Autodesk Inventor part; units mm, degrees
ref_plane "YZ Plane" through (0, 0, 0) normal (1, 0, 0) x (0, 1, 0)
ref_plane "XZ Plane" through (0, 0, 0) normal (0, 1, 0) x (-1, 0, 0)
ref_plane "XY Plane" through (0, 0, 0) normal (0, 0, 1) x (1, 0, 0)
sketch "Sketch1" plane through (0, 0, 0) normal (0, 1, 0) x (-1, 0, 0)
  line L0 (0, 0) -> (0, -8)
  circle A0 centre (0, -8) radius 3
  line L1 (0, 0) -> (0, 8)
  circle A1 centre (0, 8) radius 2.5
  circle A2 centre (0, 8) radius 3.75
  circle A3 centre (0, -8) radius 3.75
  line L2 (3.75, 8) -> (3.75, -8)
  line L3 (-3.75, 8) -> (-3.75, -8)
  line L4 (3.75, 4.25) -> (-3.75, 4.25)
  line L5 (3.75, -4.25) -> (-3.75, -4.25)
  point P0 (-2.6582, -4.25)
  dimension "d0" = 8
  dimension "d1" = 6
  dimension "d2" = 8
  dimension "d3" = 5
  dimension "d4" = 7.5
  dimension "d5" = 7.5
  dimension "d6" = 8.5
extrude "Extrusion1" add sketch "Sketch1" along normal blind 5 contours L1 L4 L2 L5 L0 | L0 L5 L3 L4 L1 | L4 L3 A2 | A2 | A2 L2 L4
sketch "Sketch2" plane through (3.75, 0, -4.25) normal (0, 0, -1) x (-1, 0, 0)
  line L0 (0, 5) -> (7.5, 5)
  line L1 (0, 0) -> (7.5, 0)
  line L2 (7.5, 0) -> (7.5, 5)
  line L3 (7.5, 5) -> (0, 5)
  line L4 (0, 5) -> (0, 0)
  line L5 (0, 0) -> (7.5, 5) construction
  line L6 (7.5, 0) -> (0, 5) construction
  circle A0 centre (3.75, 2.5) radius 1.5
  line L7 (1.25, 1.5) -> (6.25, 1.5)
  line L8 (6.25, 1.5) -> (6.25, 3.5)
  line L9 (6.25, 3.5) -> (1.25, 3.5)
  line L10 (1.25, 3.5) -> (1.25, 1.5)
  line L11 (1.25, 1.5) -> (6.25, 3.5) construction
  line L12 (6.25, 1.5) -> (1.25, 3.5) construction
  point P0 (3.75, 0)
  point P1 (4.868, 1.5)
  point P2 (2.632, 1.5)
  point P3 (2.632, 3.5)
  point P4 (4.868, 3.5)
  dimension "d9" = 3
  dimension "d10" = 5
  dimension "d11" = 2
extrude "Extrusion2" cut sketch "Sketch2" against normal blind 8.5
sketch "Sketch3" plane through (3.75, 0, 8) normal (1, 0, 0) x (0, 0, -1)
  line L0 (0, 0) -> (0, 5)
  circle A0 centre (0, 2.5) radius 1.5
  point P0 (8, 0)
  dimension "d14" = 3
extrude "Extrusion3" add sketch "Sketch3" along normal mid plane 1.5
sketch "Sketch4" plane through (4.5, 2.5, 8) normal (1, 0, 0) x (0, 0, -1)
  line L0 (0, -2.5) -> (0, 2.5)
  circle A0 centre (0, 0) radius 1
  point P0 (8, -2.5)
  dimension "d17" = 2
extrude "Extrusion4" cut sketch "Sketch4" against normal blind 3.2625
properties part number "Link_InsideV3"
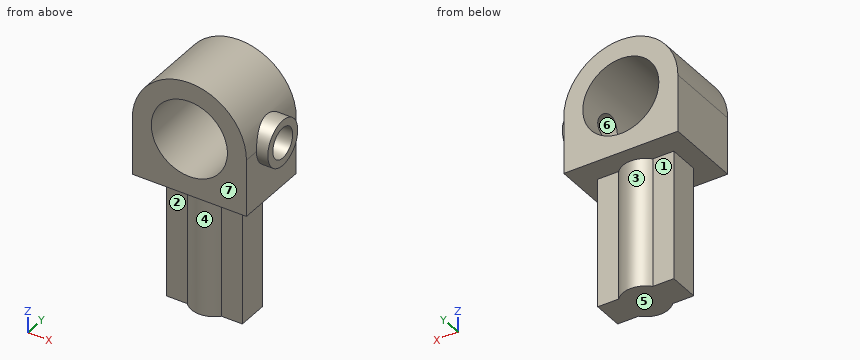
Input: part model. Units: mm. Frame: model coordinates. Face numbers are marked on the shaded views. A direction names the side the tool comes from. Give positions to 0.01 mm unless a question says otherwise; leave off trailing zeros. Order: outer loops, then holes, each group sorted by start corner. A loop starts at its lowest first (then second) coordinate and runs counter-clockwise, first axis right, second up.
1. Draft query along Z for the marked faces 5, 6 and 7. Return one class per face: released by +Z, released by -Z, zero draft, split by the parting line, or undercut.
Computed:
face 5: released by -Z
face 6: undercut
face 7: zero draft
2. Pin query (flat end, axial travel): pin 1 Ø1.1 at (x, z) = (-2, -2) entering from +Y; pin 2 Ø1 at (y, z) = (2, 0.5) entering from -X; pin 3 Ø0.6 at (y, z) = (3, 2) entering from +X. Return the tip coordinate at first contact, or that it passes through.
Computed:
pin 1: stops at y = 3.5
pin 2: stops at x = -2.5
pin 3: stops at x = 2.5
3. Cut plane A-A (x = 0). Return loops of the section in (y, z), and give its area (3 significant figures).
Computed:
outline: (0, 4.25) - (1, 4.25) - (1, -4.25) - (4, -4.25) - (4, 4.25) - (5, 4.25) - (5, 5.5) - (0, 5.5) - close; (0, 10.5) - (5, 10.5) - (5, 11.75) - (0, 11.75) - close
area: 38.0 mm2
4. Cut plane D-D (y = 2.5). Return loops of the section in (x, z), and give its area (3 significant figures).
Computed:
outline: (-3.75, 4.25) - (-2.5, 4.25) - (-2.5, -4.25) - (2.5, -4.25) - (2.5, 4.25) - (3.75, 4.25) - (3.75, 6.5) - (4.5, 6.5) - (4.5, 7) - (2.29, 7) arc R2.5 cw (long way) to (2.29, 9) - (4.5, 9) - (4.5, 9.5) - (3.44, 9.5) arc R3.75 ccw to (-3.75, 8) - close
area: 71.3 mm2
5. Cut plane B-B (z = 2.5). Return loops of the section in (x, y), and give its area (3 significant figures).
Computed:
outline: (-2.5, 1.5) - (-1.12, 1.5) arc R1.5 ccw to (1.12, 1.5) - (2.5, 1.5) - (2.5, 3.5) - (1.12, 3.5) arc R1.5 ccw to (-1.12, 3.5) - (-2.5, 3.5) - close
area: 11.5 mm2
6. Cut plane C-C (x = 3). Return loops of the section in (y, z), and give its area (3 significant figures).
Computed:
outline: (0, 4.25) - (5, 4.25) - (5, 10.25) - (0, 10.25) - close; hole circle Ø2 at (2.5, 8)
area: 26.9 mm2
7. Line query: probe 1 along Z at (x, y) = (0, 2.55); probe 2 along Y at (x, z) = (3.1, 8); probe 3 along Z at (x, y) = (4.05, 2.5). Output: solid intervals per line, ascending.
Computed:
probe 1: z = -4.25 to 5.5, 10.5 to 11.75
probe 2: y = 0 to 1.5, 3.5 to 5
probe 3: z = 6.5 to 7, 9 to 9.5
8. Set-up query: the marked faces 1, 2, 3 and 4. Return all of +Z, -Z, +X, -X, +Y, -Y with unobstructed straight access to the full face (end or side cutting, diameter ignored); none if empty.
Computed:
face 1: -Z, -X, +Y
face 2: -Z, -X, -Y
face 3: -Z, +Y
face 4: -Z, -Y
